```python
from build123d import *

# Parameters (mm, degrees)
ESQUISSE1_R             = 3
BOSS_EXTRU_1_DEPTH      = 60
ESQUISSE2_R             = 5
BOSS_EXTRU_2_DEPTH      = 6
ENL_V_MAT_EXTRU_1_DEPTH = 4.5


with BuildPart() as part:
    # Esquisse1 → Boss.-Extru.1 (new body)
    with BuildSketch(Plane.XY):
        Circle(ESQUISSE1_R)
    extrude(amount=BOSS_EXTRU_1_DEPTH)

    # Esquisse2 → Boss.-Extru.2 (add)
    with BuildSketch(Plane.XY.offset(60)):
        Circle(ESQUISSE2_R)
    extrude(amount=BOSS_EXTRU_2_DEPTH)

    # Esquisse3 → Enlèv. mat.-Extru.1 (cut)
    with BuildSketch(Plane.XY.offset(66)):
        Polygon((4.041451884, 0), (2.020725942, 3.5), (-2.020725942, 3.5), (-4.041451884, 0), (-2.020725942, -3.5), (2.020725942, -3.5), align=None)
    extrude(amount=-ENL_V_MAT_EXTRU_1_DEPTH, mode=Mode.SUBTRACT)


solid = part.part
```
Input: part model. Units: mm. Frame: model coordinates. A direction names the side the tool comes from. Coordinates: 2 decimals unless noted, no trailing zeros. Write each loop counter-clockwise with the first axis right and the second up, starting at its lowest first coordinate (ties: lowest second). Pieces come first, ordered by that corner, then holes. Notation, with made-up numbers: (79, 32) - (138, 32) arc R7 ccw to (138, 39) - close; hole circle Ø8 at (-3.75, 16). An arc over 180 degrees is marked (long way). Put each result on its own line as item: value. Start each with the question number.
1) Contact query for flat-ended pins moving along their axis: pin 1 (3 mm diameter, centred on x = -3.5, z = 57, fed in from +Y); pin 2 (2 mm diameter, centred on x = 2, y = 2.5, fed in from -Z); pin 3 (1 mm diameter, centred on x = 1, y = -1, fed in from +Z); pin 4 (6 mm diameter, centred on y = 3, z = 22.5, fed in from -X). Output: stop coordinate, or through.
2) Ray query, L1, parallel to Z at x = -1.75, y = 1.75; L2, parallel to Y at x = 0, z = 7; L3, parallel to Z at x = -3.25, y = 1.25. Return the intervals inside material, ascending.
3) Reachability of faces 4 (the face through (-3, 0, 30)), 5 (the face through (-3.045, -1.726, 63.782)), 6 (the face through (0, -4, 66)) from +Z, -Z, +X, -X, +Y, -Y: full face, straight path, thin tool, end or side. Return the list, or none.
4) Mould query, pull axis Y, two halves, no side actions, for faces 1 (the face through (3, -1.8, 63.8)), 2 (the face through (-0.1, -3.3, 60)), 3 (the face through (-1.08, -4.88, 62.96)). Classes: pulls with the +Y half, pulls with the -Y half, needs draft (parallel to the pull), parting line crosses it, or undercut.
5) Cut plane A-A (x = 0). Return the cut outline in (y, z).
6) Cut plane B-B (z = 6). Return the cut outline in (x, y), plus the area to 3 significant figures.
7) Cut plane C-C (y = 1). Return the cut outline in (x, z).
Resolved:
1. pin 1: stops at y = 2.24
1. pin 2: stops at z = 0
1. pin 3: stops at z = 61.5
1. pin 4: stops at x = -3
2. L1: z = 0 to 61.5
2. L2: y = -3 to 3
2. L3: z = 60 to 61.5
3. face 4: -Z
3. face 5: +Z
3. face 6: +Z, +X, -X, +Y, -Y
4. face 1: undercut
4. face 2: needs draft
4. face 3: parting line crosses it
5. outline: (-5, 60) - (-3, 60) - (-3, 0) - (3, 0) - (3, 60) - (5, 60) - (5, 66) - (3.5, 66) - (3.5, 61.5) - (-3.5, 61.5) - (-3.5, 66) - (-5, 66) - close
6. outline: circle Ø6 at (0, 0)
6. area: 28.3 mm2
7. outline: (-4.9, 60) - (-2.83, 60) - (-2.83, 0) - (2.83, 0) - (2.83, 60) - (4.9, 60) - (4.9, 66) - (3.46, 66) - (3.46, 61.5) - (-3.46, 61.5) - (-3.46, 66) - (-4.9, 66) - close
